from build123d import *

# Parameters (mm, degrees)
F0_R     = 11
F1_DEPTH = 7
F2_DEPTH = 7


# Not quite as in the source:
# - a feature names something its author has since deleted; it is built from what else it names


with BuildPart() as f1:
    # F0 (on Top) → F1 (new body)
    with BuildSketch(Plane.XY):
        with BuildLine():
            ThreePointArc((29.3501442774, 1.4728811124), (17.7035935394, 9.3195381001), (16.7314646223, 23.3290753994))
            ThreePointArc((16.7314646223, 23.3290753994), (0, 18.0157402468), (-16.7314646223, 23.3290753994))
            ThreePointArc((-16.7314646223, 23.3290753994), (-15.8555966996, 20.3808641164), (-15.56, 17.3195381001))
            ThreePointArc((-15.56, 17.3195381001), (-19.4902507988, 6.8161503505), (-29.3501442774, 1.4728811124))
            ThreePointArc((-29.3501442774, 1.4728811124), (-16.8351135056, -10.0081099666), (-12.8952216464, -26.5282916699))
            ThreePointArc((-12.8952216464, -26.5282916699), (-0.0001071921, -20.0000000004), (12.8950947338, -26.5281188876))
            ThreePointArc((12.8950947338, -26.5281188876), (16.8350899961, -10.0080120701), (29.3501442774, 1.4728811124))
        make_face()
        Circle(F0_R, mode=Mode.SUBTRACT)
    extrude(amount=F1_DEPTH)

    # F0 (on Top) → F2 (join)
    with BuildSketch(Plane.XY):
        with BuildLine():
            ThreePointArc((29.3501442774, 1.4728811124), (42.0633877496, 5.2497888988), (47.56, 17.3195381001))
            ThreePointArc((47.56, 17.3195381001), (34.6213260163, 33.0239414005), (16.7314646223, 23.3290753994))
            ThreePointArc((16.7314646223, 23.3290753994), (17.7035935394, 9.3195381001), (29.3501442774, 1.4728811124))
        make_face()
        with Locations((31.56, 17.3195381001)):
            Circle(F0_R, mode=Mode.SUBTRACT)
        with BuildLine():
            ThreePointArc((-15.56, 17.3195381001), (-15.8555966996, 20.3808641164), (-16.7314646223, 23.3290753994))
            ThreePointArc((-16.7314646223, 23.3290753994), (-42.6554805123, 28.8473441446), (-38.1316823001, 2.7314267848))
            ThreePointArc((-38.1316823001, 2.7314267848), (-33.8298826127, 1.4813679746), (-29.3501442774, 1.4728811124))
            ThreePointArc((-29.3501442774, 1.4728811124), (-19.4902507988, 6.8161503505), (-15.56, 17.3195381001))
        make_face()
        with Locations((-31.56, 17.3195381001)):
            Circle(F0_R, mode=Mode.SUBTRACT)
        with BuildLine():
            ThreePointArc((16, -36), (15.2039717794, -31.0161017135), (12.8950947338, -26.5281188876))
            ThreePointArc((12.8950947338, -26.5281188876), (-0.0001071921, -20.0000000004), (-12.8952216464, -26.5282916699))
            ThreePointArc((-12.8952216464, -26.5282916699), (-4.9837964273, -51.2040051687), (16, -36))
        make_face()
        with Locations((0, -36)):
            Circle(F0_R, mode=Mode.SUBTRACT)
    extrude(amount=F2_DEPTH)


solid = f1.part
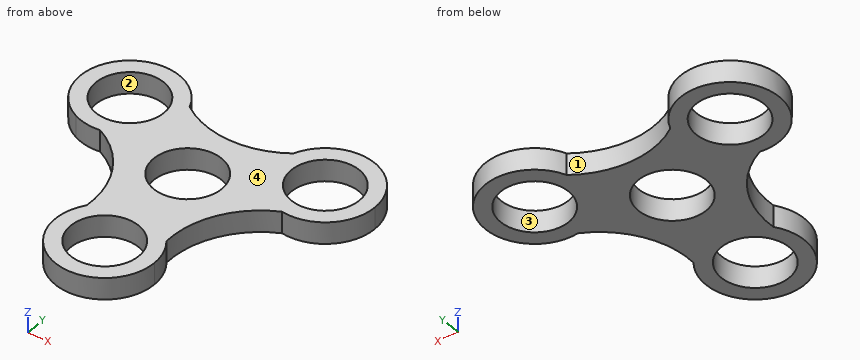
Geometry: final body of the model. Coordinates: model frame, mm. Face numbers are marked on the shaded views. Coordinates: 2 decimals unless noted, no trailing zeros. Loops run counter-clockwise (first coordinate to the right, second up) from the corner with the lowest first, then second, coordinate; pieces in that order, holes last. Notation, with made-up numbers: (34, 65) - (39, 65) arc R6 ccw to (39, 73) - close; hole circle Ø5 at (45.5, 3). An arc over 180 degrees is marked (long way). Put each result on its own line as item: value. Start each with the question number.
Q1. Line query: line 1 (Y direction, x = 0, z = 1.75); line 2 (Y direction, x = 31.56, z = 3.75); line 3 (Y direction, x = 10, z = 6.75). Output: solid intervals per line, ascending.
Q2. Cut plane D-D, the plane y = 0. Return loops of the section in (x, z).
Q3. Cut plane C-C, the plane x = 33.5. Return loops of the section in (y, z), and give its area (3 significant figures).
Q4. Pull-direction query (Y, two-part tool) for the marked faces 1, 2, 3 and 4; classes: released by +Y, released by -Y, zero draft, split by the parting line, or undercut.
Q5. Cut plane B-B, the plane y = 14.5. Return loops of the section in (x, z), and give its area (3 significant figures).
Q6. Cut plane A-A, the plane x = 0. Return loops of the section in (y, z), and give its area (3 significant figures).
Q7. Pin query (flat end, axial travel): pin 1 Ø4 at (y, z) = (-35, 1) entering from -X; pin 2 Ø3 at (y, z) = (19, 4) entering from -X; pin 3 Ø1.5 at (x, z) = (-20.5, 2.5) entering from -Y. Return the tip coordinate at first contact, or that it passes through.
Filled sheet:
1. line 1: -52 to -47, -25 to -11, 11 to 18.02
1. line 2: 1.32 to 6.32, 28.32 to 33.32
1. line 3: -48.49 to -40.58, -31.42 to -4.58, 4.58 to 19.79
2. outline: (-26.64, 0) - (-11, 0) - (-11, 7) - (-26.64, 7) - close; (11, 0) - (26.64, 0) - (26.64, 7) - (11, 7) - close
3. outline: (1.44, 0) - (6.49, 0) - (6.49, 7) - (1.44, 7) - close; (28.15, 0) - (33.2, 0) - (33.2, 7) - (28.15, 7) - close
3. area: 70.8 mm²
4. face 1: released by +Y
4. face 2: undercut
4. face 3: undercut
4. face 4: zero draft
5. outline: (-47.31, 0) - (-42.19, 0) - (-42.19, 7) - (-47.31, 7) - close; (-20.93, 0) - (20.93, 0) - (20.93, 7) - (-20.93, 7) - close; (42.19, 0) - (47.31, 0) - (47.31, 7) - (42.19, 7) - close
5. area: 365 mm²
6. outline: (-52, 0) - (-47, 0) - (-47, 7) - (-52, 7) - close; (-25, 0) - (-11, 0) - (-11, 7) - (-25, 7) - close; (11, 0) - (18.02, 0) - (18.02, 7) - (11, 7) - close
6. area: 182 mm²
7. pin 1: x = -16
7. pin 2: x = -47.56
7. pin 3: y = -5.91
